Geometry: see drawing. Coordinates: mm, zero at the bounding-box minimum. A direction names the side the tool comes from. Coordinates: 2 decimals unless noted, no trailing zeros. Write each loop counter-clockwise with the first axis right and the second up, starting at its lowest first coordinate (ties: lowest second). Pieces come first, ordered by that corner, then holes. Notation, with made-up numbers: (85.25, 84.25) - (115.25, 84.25) arc R21 ccw to (115.25, 104.25) - close; hole circle Ø5 at (64.5, 28). An arc over 180 degrees is marked (long way). Use a Markdown table: item, result. Add a question column.
Q1. Material intervals for probe 1 along Z at (x, y) = (257.5, 18); probe 2 along Z at (x, y) = (150, 4.75); probe 3 along X at (y, z) = (9, 75), sorted ascending. Write a range as from..to.
Q2. Section query A-A (x = 234). Return the cut outline in (y, z), then the cut area to 3 significant figures.
Q3. Set-up query: the marked faces 4, 5, 6 and 7. Return all of +Z, -Z, +X, -X, +Y, -Y with unobstructed straight access to the full face (end or side cutting, diameter ignored); none if empty.
Q4. Section query C-C (z = 75). Return the cut outline in (x, y).
Q5. Mould query, pull axis X, two halves, no side actions, for the marked faces 1, 2 and 3. Classes: released by +X, released by -X, zero draft, split by the parting line, or undercut.
Q6. Pin query (flat end, axial travel): P1, Ø10, axis at x = 46, y = 7, coming from the +Z side; P2, Ø10, axis at x = 43, y = 7.5, coming from the -Z side; P3, Ø1.5, axis at y = 8.5, z = 75, coming from the -X side. Return the tip coordinate at first contact, or that it passes through.
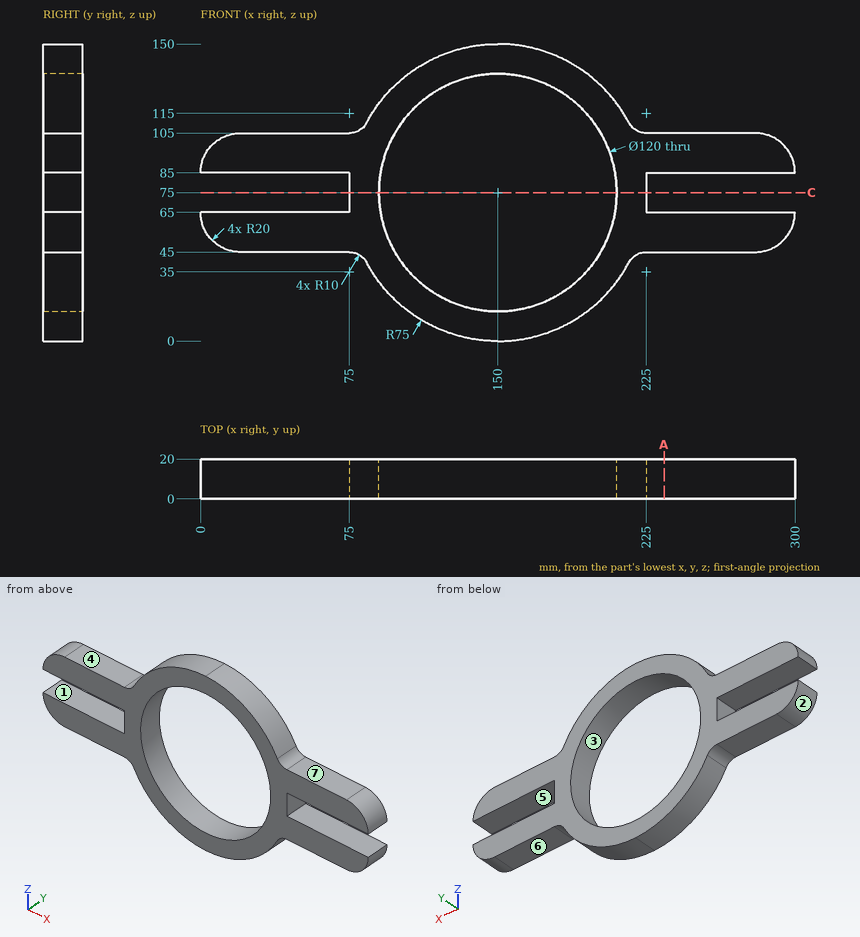
Values follow:
| question | item | result |
|---|---|---|
| 1 | probe 1 | 45..65, 85..105 |
| 1 | probe 2 | 0..15, 135..150 |
| 1 | probe 3 | 75..90, 210..225 |
| 2 | outline | (0, 45) - (20, 45) - (20, 65) - (0, 65) - close; (0, 85) - (20, 85) - (20, 105) - (0, 105) - close |
| 2 | area | 800 mm2 |
| 3 | face 4 | +Z, -X, +Y, -Y |
| 3 | face 5 | +X, +Y, -Y |
| 3 | face 6 | -Z, +X, +Y, -Y |
| 3 | face 7 | +Z, +X, +Y, -Y |
| 4 | outline | (75, 0) - (90, 0) - (90, 20) - (75, 20) - close; (210, 0) - (225, 0) - (225, 20) - (210, 20) - close |
| 5 | face 1 | zero draft |
| 5 | face 2 | released by -X |
| 5 | face 3 | undercut |
| 6 | P1 | z = 105 |
| 6 | P2 | z = 45 |
| 6 | P3 | x = 75 |
